The listing builds one solid part. Answer for the finished solid, in the listing's coordinates (mm). A direction names the side the tool comes from. Round coordinates to 2 decimals unless told otherwise and drop trailing zeros. Write each loop counter-clockwise with the first axis right and the second up, starting at its lowest first coordinate (ties: lowest second). Pieces come first, ordered by that corner, then holes. Notation, with made-up numbers: M 41,25.5 L 84,25.5 A27 cw 84,47.5 Z; hole C 9.5,82 d1. An arc over 180 degrees is marked long. Write each question's results on one line, items separated by ' | '.
Autodesk Inventor part; units mm, degrees
ref_plane "YZ Plane" through (0, 0, 0) normal (1, 0, 0) x (0, 1, 0)
ref_plane "XZ Plane" through (0, 0, 0) normal (0, 1, 0) x (-1, 0, 0)
ref_plane "XY Plane" through (0, 0, 0) normal (0, 0, 1) x (1, 0, 0)
sketch "Sketch1" plane through (0, 0, 0) normal (0, 0, 1) x (1, 0, 0)
  point P0 (0, 0)
sketch "Sketch2" plane through (0, 0, 0) normal (0, 0, 1) x (1, 0, 0)
  line L0 (0, 0) -> (250, 0)
  line L1 (250, 0) -> (250, 250)
  line L2 (250, 250) -> (0, 250)
  line L3 (0, 250) -> (0, 0)
  line L4 (0, 0) -> (-70, 0)
  line L5 (-70, 0) -> (0, 70)
  dimension "d0" = 250
  dimension "d1" = 250
  dimension "d2" = 70
  dimension "d3" = 45
extrude "Extrusion1" add sketch "Sketch2" along normal blind 142
sketch "Sketch3" plane through (0, 0, 142) normal (0, 0, 1) x (1, 0, 0)
  line L0 (4, 3) -> (180, 3)
  line L1 (-70, 0) -> (250, 0)
  line L2 (4, 3) -> (180, 3) construction
  line L3 (180, 3) -> (180, 246)
  line L4 (4, 3) -> (4, 246)
  line L5 (4, 3) -> (247, 3) construction
  line L6 (250, 250) -> (0, 250)
  line L7 (4, 246) -> (180, 246)
  point P0 (0, 0)
  dimension "d6" = 176
  dimension "d7" = 0
  dimension "d8" = 243
  dimension "d9" = 243
  dimension "d10" = 90
extrude "Extrusion2" cut sketch "Sketch3" against normal blind 135
sketch "Sketch4" plane through (4, 3, 142) normal (0, 1, 0) x (1, 0, 0)
  line L0 (3, 3) -> (173, 3)
  line L1 (176, 0) -> (0, 0)
  line L2 (173, 3) -> (173, 132)
  line L3 (173, 132) -> (3, 132)
  line L4 (176, 135) -> (0, 135)
  line L5 (3, 132) -> (3, 3)
  line L6 (176, 0) -> (176, 135)
  line L7 (0, 0) -> (0, 135)
  point P0 (-4, 142)
  dimension "d13" = 3
  dimension "d14" = 3
  dimension "d15" = 3
  dimension "d16" = 3
extrude "Extrusion3" cut sketch "Sketch4" against normal through all contours L5 L3 L2 L0
sketch "Sketch5" plane through (4, 3, 142) normal (0, 1, 0) x (1, 0, 0)
  line L0 (176, 0) -> (0, 0)
  line L1 (0, 0) -> (0, 3)
  line L2 (3, 3) -> (3, 132)
  line L3 (0, 3) -> (176, 3)
  line L4 (176, 0) -> (176, 135)
  line L5 (176, 0) -> (0, 0)
  line L6 (3, 3) -> (173, 3)
  point P0 (-4, 142)
extrude "Extrusion4" add sketch "Sketch5" along normal blind 7
sketch "Sketch6" plane through (-70, 0, 0) normal (0, -1, 0) x (1, 0, 0)
  line L0 (315, 137) -> (254, 137)
  line L1 (254, 137) -> (254, 5)
  line L2 (254, 5) -> (315, 5)
  line L3 (315, 5) -> (315, 137)
  line L4 (0, 142) -> (320, 142)
  line L5 (0, 0) -> (320, 0)
  line L6 (320, 0) -> (320, 142)
  line L7 (247, 139) -> (247, 10)
  point P0 (70, 0)
  dimension "d21" = 5
  dimension "d22" = 5
  dimension "d23" = 5
  dimension "d24" = 7
extrude "Extrusion5" cut sketch "Sketch6" against normal blind 246
sketch "Sketch7" plane through (-70, 0, 0) normal (0, -1, 0) x (1, 0, 0)
  line L0 (254, 5) -> (254, 137)
  line L1 (315, 137) -> (315, 5)
  line L2 (254, 137) -> (315, 137)
  line L3 (315, 137) -> (315, 5)
  line L4 (315, 5) -> (254, 5)
  line L5 (254, 5) -> (254, 137)
  point P0 (70, 0)
  point P1 (315, 5)
extrude "Extrusion6" add sketch "Sketch7" against normal blind 10
properties part number "Body_updated"
1) Find the intervals of material crossed by line 1 (X direction, y = 202.5, z = 93); line 2 (Y direction, x = 6, z = 132); line 3 (Z direction, x = 221, y = 150), in increasing order.
Return value:
line 1: 0 to 4, 180 to 184, 245 to 250 | line 2: 0 to 3, 246 to 250 | line 3: 0 to 5, 137 to 142
2) Section B-B (y = 81) is taken. Determine the outline of the cut face in (x, z), then the cut area to 3 significant figures.
Return value:
outline: M 0,0 L 250,0 L 250,142 L 180,142 L 180,7 L 4,7 L 4,142 L 0,142 Z; hole M 184,5 L 245,5 L 245,137 L 184,137 Z | area: 3,690 mm²
3) Section C-C (z = 51.5) is taken. Determine the outline of the cut face in (x, y), then the cut area to 3 significant figures.
Return value:
outline: M -70,0 L 7,0 L 7,3 L 4,3 L 4,246 L 180,246 L 180,3 L 177,3 L 177,0 L 250,0 L 250,250 L 0,250 L 0,70 Z; hole M 184,10 L 245,10 L 245,246 L 184,246 Z | area: 7,280 mm²
4) The mould has two halves that part along X. Classify faces 1 (the face through (250, 123, 70)), 2 (the face through (180, 123, 75)), 3 (the face through (-35, 35, 70)), 4 (the face through (91, 246, 75)): +X half, -X half, draft (parallel to the pull), parting line (faces both ways), or undercut.
Return value:
face 1: +X half | face 2: undercut | face 3: -X half | face 4: undercut
5) A tool of negligible diameter and unlimited length cuts with its end or side. For faces 5 (the face through (88, 0, 9)), 6 (the face through (0, 161, 70)), 7 (the face through (214, 10, 72)), from which of +Z, -Z, +X, -X, +Y, -Y can it reach the whole face along a straight path? Write none if from no direction.
Return value:
face 5: +Z, -Z, +X, -X, -Y | face 6: +Z, -Z, -X, +Y | face 7: none
6) Section A-A (x = 148.5) is taken. Determine the outline of the cut face in (y, z), then the cut area to 3 significant figures.
Return value:
outline: M 0,0 L 250,0 L 250,142 L 246,142 L 246,7 L 3,7 L 3,10 L 0,10 Z; M 0,139 L 10,139 L 10,142 L 0,142 Z | area: 2,330 mm²
7) Section D-D (x = -23.5) is taken. Determine the outline of the cut face in (y, z), then the cut area to 3 significant figures.
Return value:
outline: M 0,0 L 46.5,0 L 46.5,142 L 0,142 Z | area: 6,600 mm²
8) Each of these flat-tipped pins is pushed along its axis until it touches: pin 1 (3.5 mm diameter, centred on y = 1.5, z = 43, fed in from -X); pin 2 (10 mm diameter, centred on y = 39.5, z = 39, fed in from -X); pin 3 (2 mm diameter, centred on x = -36, z = 83.5, fed in from +Y). Where does it stop, or does it pass through?
Return value:
pin 1: x = -70 | pin 2: x = -35.5 | pin 3: y = 35
